from build123d import *

# Parameters (mm, degrees)
AUFSATZ_LINEAR_AUSTRAGEN1_DEPTH                      = 19
AUFSATZ_LINEAR_AUSTRAGEN1_DEPTH_BACK                 = 19
STIRNSENKUNG_F_R_M2_FLACHKOPFSCHRAUBE_MI_D           = 2.4
STIRNSENKUNG_F_R_M2_FLACHKOPFSCHRAUBE_MI_CBORE_D     = 5
STIRNSENKUNG_F_R_M2_FLACHKOPFSCHRAUBE_MI_CBORE_DEPTH = 1.6
FASE1_SIZE                                           = 2


with BuildPart() as part:
    # Skizze1 → Aufsatz-Linear austragen1 (new, two sides: drawn at the far end of the back side and taken through both)
    with BuildSketch(Plane.XY.offset(-AUFSATZ_LINEAR_AUSTRAGEN1_DEPTH_BACK)):
        Polygon((-3.5, 0), (-3.5, 3), (-6.5, 3), (-6.5, 6.5), (6.5, 6.5), (6.5, 3), (3.5, 3), (3.5, 0), (13.5, 0), (13.5, 10.8), (-13.5, 10.8), (-13.5, 0), align=None)
    extrude(amount=AUFSATZ_LINEAR_AUSTRAGEN1_DEPTH + AUFSATZ_LINEAR_AUSTRAGEN1_DEPTH_BACK)

    # Stirnsenkung für M2 Flachkopfschraube mit Schlitz1 (through all)
    with Locations(Plane(origin=(0, 0, 0), x_dir=(-1, 0, 0), z_dir=(0, -1, 0))):
        with Locations((-10, -7.5), (-10, 7.5), (10, -7.5), (10, 7.5)):
            CounterBoreHole(STIRNSENKUNG_F_R_M2_FLACHKOPFSCHRAUBE_MI_D / 2, STIRNSENKUNG_F_R_M2_FLACHKOPFSCHRAUBE_MI_CBORE_D / 2, STIRNSENKUNG_F_R_M2_FLACHKOPFSCHRAUBE_MI_CBORE_DEPTH)

    # Fase1
    # the kernel refuses this chamfer: 2 mm, written as the material it takes off along each edge
    with BuildSketch(Plane(origin=(-13.5, 0, 24.143365976), x_dir=(0.9996219169112968, -0.027495876610586598, 0), z_dir=(0, 0, -1)), Plane(origin=(13.5, 0, -24.143365976), x_dir=(-0.9996219169112968, -0.027495876610586608, 0), z_dir=(0, 0, 1))) as fase1_piece_1:
        Polygon((FASE1_SIZE * 0.999621916911, -FASE1_SIZE * 0.0274958766106), (-FASE1_SIZE * 0.0274958766106, -FASE1_SIZE * 0.999621916911), (0, 0), align=None)
    extrude(amount=48.286731952, mode=Mode.SUBTRACT)


solid = part.part
Build history of the part. All positions in model axes, mm. A direction names the side the tool comes from. Coordinates: 2 decimals unless noted, no trailing zeros. Order: outer loops, then holes, each group sorted by start corner. A loop starts at its lowest first (then second) coordinate and runs counter-clockwise, first axis right, second up. Notation, with made-up numbers: M -14.5,30.25 L 34.5,30.25 A15 cw 34.5,54.25 Z; hole C 51.5,0 d9. An arc over 180 degrees is marked long. One line per question, with ' | ' between items. Start each with the question number.
Q1. Saw through at A-A (y = 4.25). List the corners of the cut face in (x, z).
Q2. Saw through at C-C (x = 10). List the corners of the cut face in (y, z), then the cut area to 3 significant figures.
Q3. Two-plate mould, pull along Z, no slides. Class faces 5 (the face through (0, 10.8, 0)), 6 (the face through (-9, 1.6, 9)), 7 (the face through (9.84, 6.26, 6.31)): +Z half, -Z half, draft (parallel to the pull), parting line (faces both ways), or undercut.
Q4. Probe L1, parallel to X at y = 8, z = -7.5; L2, parallel to Z at x = -10, y = 1.3; L3, parallel to Z at x = -10, y = 5.25. List the from-to ranges inside material, lowest first. Write a range as from..to.
Q5. Flat gauge pins, fed straight in: pin 1 Ø6.5 at (x, z) = (-10, 7.5) entering from +Y; pin 2 Ø1.5 at (x, z) = (11, 6.5) entering from -Y; pin 3 Ø5 at (x, z) = (0.5, -0.5) entering from -Y. Where does each tip first touch, or does it go through?
Q6. 3-axis set-ups, long thin cutter, end or side, ignore diameter. For faces 1 (the face through (11, 1.6, 9)), 2 (the face through (-3.5, 1, 0)), 3 (the face through (6.5, 5, 0)), 4 (the face through (10.65, 6.26, -8.51)): which of +Z, -Z, +X, -X, +Y, -Y reach the whole face in a straight line?
Q7. Saw through at D-D (x = -4.25). List the corners of the cut face in (y, z).
Q8. Saw through at B-B (z = -7.5). List the corners of the cut face in (x, y), then the cut area to 3 significant figures.
Check values:
1) outline: M -13.5,-19 L -6.5,-19 L -6.5,19 L -13.5,19 Z; M 6.5,-19 L 13.5,-19 L 13.5,19 L 6.5,19 Z; hole C -10,-7.5 d2.4; hole C -10,7.5 d2.4; hole C 10,-7.5 d2.4; hole C 10,7.5 d2.4
2) outline: M 0,-19 L 10.8,-19 L 10.8,-8.7 L 1.6,-8.7 L 1.6,-10 L 0,-10 Z; M 0,-5 L 1.6,-5 L 1.6,-6.3 L 10.8,-6.3 L 10.8,6.3 L 1.6,6.3 L 1.6,5 L 0,5 Z; M 0,10 L 1.6,10 L 1.6,8.7 L 10.8,8.7 L 10.8,19 L 0,19 Z | area: 350 mm2
3) face 5: draft | face 6: undercut | face 7: undercut
4) L1: x = -13.5..-11.2, -8.8..8.8, 11.2..13.5 | L2: z = -19..-10, -5..5, 10..19 | L3: z = -19..-8.7, -6.3..6.3, 8.7..19
5) pin 1: stops at y = 10.8 | pin 2: stops at y = 1.6 | pin 3: stops at y = 6.5
6) face 1: -Y | face 2: +Z, -Z, -Y | face 3: +Z, -Z | face 4: +Y, -Y
7) outline: M 0,-19 L 3,-19 L 3,19 L 0,19 Z; M 6.5,-19 L 10.8,-19 L 10.8,19 L 6.5,19 Z
8) outline: M -13.5,2 L -12.5,1 L -12.5,1.6 L -11.2,1.6 L -11.2,10.8 L -13.5,10.8 Z; M -8.8,1.6 L -7.5,1.6 L -7.5,0 L -3.5,0 L -3.5,3 L -6.5,3 L -6.5,6.5 L 6.5,6.5 L 6.5,3 L 3.5,3 L 3.5,0 L 7.5,0 L 7.5,1.6 L 8.8,1.6 L 8.8,10.8 L -8.8,10.8 Z; M 11.2,1.6 L 12.5,1.6 L 12.5,1 L 13.5,2 L 13.5,10.8 L 11.2,10.8 Z | area: 162 mm2
